Geometry: final body of the model. Coordinates: model frame, mm. Face numbers are marked on the shaded views. A direction names the side the tool comes from. Give positions to 0.01 mm unless a question says otherwise; leave off trailing zeros. Write each loop counter-clockwise with the first axis right and the second up, starting at its lowest first coordinate (ties: lowest second). Pieces come first, ordered by that corner, then holes. Notation, with made-up numbers: M 42.25,1.5 L 47.25,1.5 A24 ccw 47.25,27.5 Z; hole C 66,-17 d4. An arc over 180 degrees is marked long. Answer as a JSON object with one key per item and string values.
from build123d import *

# Parameters (mm, degrees)
SKETCH1_R           = 10
BOSS_EXTRUDE1_DEPTH = 79
FILLET1_R           = 0.5
SKETCH2_R           = 10
BOSS_EXTRUDE2_DEPTH = 2
BOSS_EXTRUDE3_DEPTH = 19.3


with BuildPart() as part:
    # Sketch1 → Boss-Extrude1 (new body)
    with BuildSketch(Plane(origin=(0, 0, 0), x_dir=(1, 0, 0), z_dir=(0, 1, 0))):
        with Locations(Location((0, 0, 0), (0, 0, 270))):
            Circle(SKETCH1_R)
    extrude(amount=BOSS_EXTRUDE1_DEPTH)

    # Fillet1
    fillet1_edges = [part.edges().sort_by_distance(p)[0] for p in [
        (0, 79, -10),
    ]]
    fillet(fillet1_edges, radius=FILLET1_R)

    # Sketch2 → Boss-Extrude2 (add)
    with BuildSketch(Plane(origin=(0, 79, 0), x_dir=(1, 0, 0), z_dir=(0, 1, 0))):
        with Locations(Location((0, 0, 0), (0, 0, 270))):
            Circle(SKETCH2_R)
    extrude(amount=BOSS_EXTRUDE2_DEPTH)

    # Sketch3 → Boss-Extrude3 (add)
    with BuildSketch(Plane(origin=(0, 81, 0), x_dir=(1, 0, 0), z_dir=(0, 1, 0))):
        with BuildLine():
            ThreePointArc((-2.7, 9.628603222), (-5.318024822, 8.468684195), (-7.5, 6.614378278))
            Line((-7.5, 6.614378278), (-7.5, -6.614378278))
            ThreePointArc((-7.5, -6.614378278), (-5.318024822, -8.468684195), (-2.7, -9.628603222))
            Line((-2.7, -9.628603222), (-2.7, 9.628603222))
        make_face()
        with BuildLine():
            ThreePointArc((7.5, 6.614378278), (5.318024822, 8.468684195), (2.7, 9.628603222))
            Line((2.7, 9.628603222), (2.7, -9.628603222))
            ThreePointArc((2.7, -9.628603222), (5.318024822, -8.468684195), (7.5, -6.614378278))
            Line((7.5, -6.614378278), (7.5, 6.614378278))
        make_face()
    extrude(amount=BOSS_EXTRUDE3_DEPTH)


solid = part.part
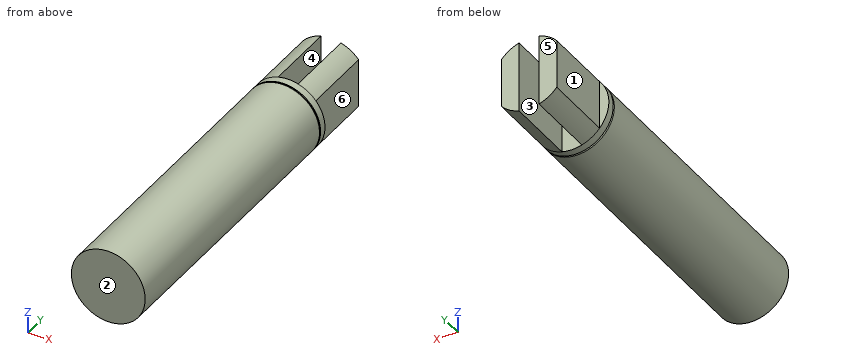
1) Cut plane C-C on y = 21. Return loops of the section in (x, z).
Geometry check:
{"outline": "C 0,0 d20"}
2) Cut plane A-A on z = 0. Return loops of the section in (x, y).
Geometry check:
{"outline": "M -10,0 L 10,0 L 10,78.5 A0.5 ccw 9.5,79 L 10,79 L 10,81 L 7.5,81 L 7.5,100.3 L 2.7,100.3 L 2.7,81 L -2.7,81 L -2.7,100.3 L -7.5,100.3 L -7.5,81 L -10,81 L -10,79 L -9.5,79 A0.5 ccw -10,78.5 Z"}
3) Set-up query: the marked faces 4, 5 and 6. Return all of +Z, -Z, +X, -X, +Y, -Y with unobstructed straight access to the full face (end or side cutting, diameter ignored); none if empty.
Geometry check:
{"face 4": "+Z, -Z, +Y", "face 5": "+Z, -Z, +X, -X, +Y", "face 6": "+Z, -Z, +X, +Y"}
4) Cut plane B-B on x = 0. Return loops of the section in (y, z).
Geometry check:
{"outline": "M 0,-10 L 78.5,-10 A0.5 ccw 79,-9.5 L 79,-10 L 81,-10 L 81,10 L 79,10 L 79,9.5 A0.5 ccw 78.5,10 L 0,10 Z"}
5) Contact query for flat-ended pins moving along their axis: P1, Ø1, axis at x = 5, y = 45.5, coming from the +Z side; P2, Ø1.3, axis at x = 9, z = -2.5, coming from the +Y side; P3, Ø1.5, axis at y = 40.5, z = -6, coming from the +X side. Output: stop coordinate, or through.
Geometry check:
{"P1": "stops at z = 8.93", "P2": "stops at y = 81", "P3": "stops at x = 8.51"}
6) Line query: line 1 (X direction, y = 96, z = -1.5); line 2 (Y direction, x = 0.5, z = 4); line 3 (X direction, y = 36, z = -7.5). Output: solid intervals per line, ascending. Write a range as from..to.
Geometry check:
{"line 1": "x = -7.5..-2.7, 2.7..7.5", "line 2": "y = 0..81", "line 3": "x = -6.61..6.61"}
7) Pull-direction query (X, two-part tool) for the marked faces 1, 2 and 3; classes: pulls with the +X half, pulls with the -X half, needs draft (parallel to the pull), parting line crosses it, or undercut.
Geometry check:
{"face 1": "pulls with the -X half", "face 2": "needs draft", "face 3": "undercut"}
